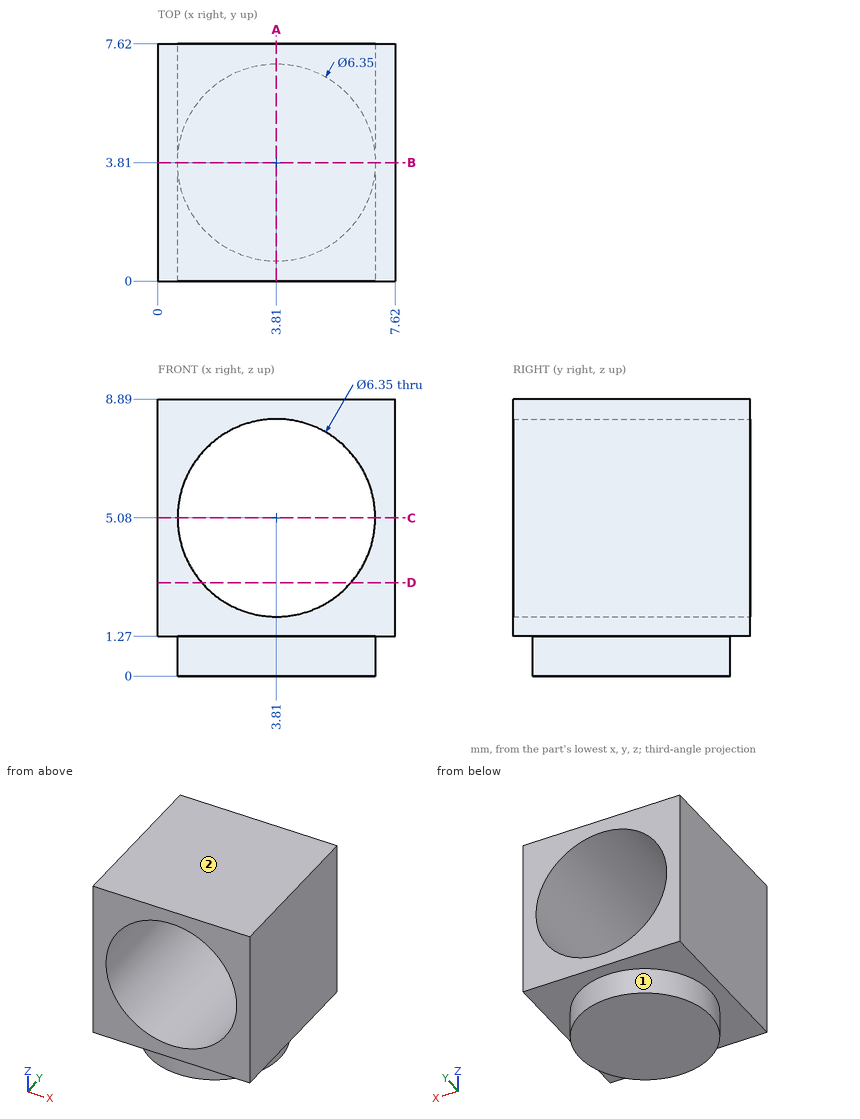
Check sheet for the drawn part. Datum: minimum x, y, z corner. Units: mm. A direction names the side the tool comes from. Give positions to 0.01 mm unless a question says otherwise; leave off trailing zeros. Order: outer loops, then holes, each group sorted by start corner. A loop starts at its lowest first (then second) coordinate and runs counter-clockwise, first axis right, second up. Notation, with made-up numbers: (14.25, 74) - (67.25, 74) arc R22 ccw to (67.25, 98) - close; hole circle Ø3 at (57, 73). An arc over 180 degrees is marked (long way). Answer in a Markdown table with one row per item. Add a question column.
Q1. Cross-section at D-D, the plane z = 3. Enter the section's corners in (x, y).
Q2. Cross-section at B-B, the plane y = 3.81. Enter the section's corners in (x, z) (3 decimals), then the cut area to 3 significant figures.
Q3. Cross-section at A-A, the plane x = 3.81. Enter the section's corners in (y, z) (3 decimals), then the cut area to 3 significant figures.
Q4. Tool access check on the marked faces 1 and 2. Record the directions out of +Z, -Z, +X, -X, +Y, -Y that give a thin tool (end or side, any length) a straight path to the whole face; none if there is none.
Q5. Material ranges on probe 1 along Z at (x, y) = (3.81, 3) (3 decimals); probe 2 along X at (y, z) = (7.5, 2.25); probe 3 along Z at (x, y) = (2.5, 3.5), recorded low to high. Write a range as from..to.
Q6. Cross-section at C-C, the plane z = 5.08. Enter the section's corners in (x, y) (3 decimals).
Check values:
| question | item | result |
|---|---|---|
| 1 | outline | (0, 0) - (1.41, 0) - (1.41, 7.62) - (0, 7.62) - close; (6.21, 0) - (7.62, 0) - (7.62, 7.62) - (6.21, 7.62) - close |
| 2 | outline | (0, 1.27) - (0.635, 1.27) - (0.635, 0) - (6.985, 0) - (6.985, 1.27) - (7.62, 1.27) - (7.62, 8.89) - (0, 8.89) - close; hole circle Ø6.35 at (3.81, 5.08) |
| 2 | area | 34.5 mm^2 |
| 3 | outline | (0, 1.27) - (0.635, 1.27) - (0.635, 0) - (6.985, 0) - (6.985, 1.27) - (7.62, 1.27) - (7.62, 1.905) - (0, 1.905) - close; (0, 8.255) - (7.62, 8.255) - (7.62, 8.89) - (0, 8.89) - close |
| 3 | area | 17.7 mm^2 |
| 4 | face 1 | -Z |
| 4 | face 2 | +Z, +X, -X, +Y, -Y |
| 5 | probe 1 | z = 0..1.905, 8.255..8.89 |
| 5 | probe 2 | x = 0..2.37, 5.25..7.62 |
| 5 | probe 3 | z = 0..2.19, 7.97..8.89 |
| 6 | outline | (0, 0) - (0.635, 0) - (0.635, 7.62) - (0, 7.62) - close; (6.985, 0) - (7.62, 0) - (7.62, 7.62) - (6.985, 7.62) - close |
